For this review, take the finished solid that the model builds, in its own axes (mm). A direction names the side the tool comes from. Round coordinates to 2 decimals unless told otherwise and drop trailing zeros. Order: outer loops, then holes, each group sorted by start corner. A loop starts at its lowest first (then second) coordinate and runs counter-clockwise, first axis right, second up. Notation, with made-up numbers: M 39.5,-39.75 L 74.5,-39.75 A21 ccw 74.5,-30.75 Z; hole C 6.5,73 d8. An arc over 180 degrees is marked long. Write item = value, one per line. Start each with the question number.
from build123d import *

# Parameters (mm, degrees)
BOX_W           = 100
BOX_H           = 63
BOX_DEPTH       = 57
PAD_DEPTH       = 60
POCKET_DEPTH    = 60
SKETCH002_R     = 8.5
POCKET001_DEPTH = 5
SKETCH003_R     = 8.5
POCKET002_DEPTH = 5
SKETCH004_R     = 8.5
POCKET003_DEPTH = 5
SKETCH005_R     = 8.5
POCKET004_DEPTH = 5
SKETCH006_R     = 8.5
POCKET005_DEPTH = 5
SKETCH007_R     = 8.5
POCKET006_DEPTH = 5
SKETCH008_W     = 12
SKETCH008_H     = 3
PAD001_DEPTH    = 12
SKETCH009_W     = 12
SKETCH009_H     = 3
PAD002_DEPTH    = 12
SKETCH010_R     = 1.6
POCKET007_DEPTH = 5


with BuildPart() as cubo:
    # Box → Box (new body)
    with BuildSketch(Plane(origin=(-50, -62, -35), x_dir=(1, 0, 0), z_dir=(0, 0, 1))):
        with Locations((50, 31.5)):
            Rectangle(BOX_W, BOX_H)
    extrude(amount=BOX_DEPTH)


with BuildPart() as cut:
    # Sketch → Pad (new body)
    with BuildSketch(Plane.XZ):
        Polygon((0, 13.1372921726), (-24.1481456572, 6.666816045), (-41.8258151869, -11.0108534847), (-48.2962913145, -35.1589991419), (-41.8258151869, -59.3071447991), (-24.1481456572, -76.9848143288), (0, -83.4552904564), (24.1481456572, -76.9848143288), (41.8258151869, -59.3071447991), (48.2962913145, -35.1589991419), (41.8258151869, -11.0108534847), (24.1481456572, 6.666816045), align=None)
    extrude(amount=PAD_DEPTH)

    # Sketch001 (on Face13 of Pad) → Pocket (cut)
    with BuildSketch(Plane(origin=(0, 0, 0), x_dir=(1, 0, 0), z_dir=(0, 1, 0))):
        Polygon((0.2789274024, 81.4748360882), (23.1696976244, 75.2404980022), (40.0320556094, 58.422596), (46.1550508689, 34.895187618), (40.0872400093, 11.9994668326), (23.2933636529, -4.8586822764), (-0.3577352301, -11.1695458715), (-23.1458968596, -4.9360655293), (-40.0016837516, 11.8309415939), (-46.2963180976, 35.1693495985), (-39.9901052234, 58.5133129971), (-22.9100181577, 75.4141328541), align=None)
    extrude(amount=-POCKET_DEPTH, mode=Mode.SUBTRACT)

    # Sketch002 (on Face11 of Pocket) → Pocket001 (cut)
    with BuildSketch(Plane(origin=(-50.566479993, 0, -50.566479993), x_dir=(0.7071067812, 0, -0.7071067812), z_dir=(-0.7071067812, 0, -0.7071067812))):
        with Locations((24.861166713, 47)):
            Circle(SKETCH002_R)
        with Locations((24.861166713, 21)):
            Circle(SKETCH002_R)
    extrude(amount=-POCKET001_DEPTH, mode=Mode.SUBTRACT)

    # Sketch003 (on Face13 of Pocket001) → Pocket002 (cut)
    with BuildSketch(Plane(origin=(-20.8638226141, 0, -77.8648460359), x_dir=(0.9659258263, 0, -0.2588190451), z_dir=(-0.2588190451, 0, -0.9659258263))):
        with Locations((9.0998185847, 47)):
            Circle(SKETCH003_R)
        with Locations((9.0998185847, 21)):
            Circle(SKETCH003_R)
    extrude(amount=-POCKET002_DEPTH, mode=Mode.SUBTRACT)

    # Sketch004 (on Face14 of Pocket002) → Pocket003 (cut)
    with BuildSketch(Plane(origin=(20.8638226141, 0, -77.8648460359), x_dir=(0.9659258263, 0, 0.2588190451), z_dir=(0.2588190451, 0, -0.9659258263))):
        with Locations((-9.0998185847, 47)):
            Circle(SKETCH004_R)
        with Locations((-9.0998185847, 21)):
            Circle(SKETCH004_R)
    extrude(amount=-POCKET003_DEPTH, mode=Mode.SUBTRACT)

    # Sketch005 (on Face12 of Pocket003) → Pocket004 (cut)
    with BuildSketch(Plane(origin=(50.566479993, 0, -50.566479993), x_dir=(0.7071067812, 0, 0.7071067812), z_dir=(0.7071067812, 0, -0.7071067812))):
        with Locations((-24.861166713, 47)):
            Circle(SKETCH005_R)
        with Locations((-24.861166713, 21)):
            Circle(SKETCH005_R)
    extrude(amount=-POCKET004_DEPTH, mode=Mode.SUBTRACT)

    # Sketch006 (on Face10 of Pocket004) → Pocket005 (cut)
    with BuildSketch(Plane(origin=(53.8508030361, 0, -14.4292791853), x_dir=(0.2588190451, 0, 0.9659258263), z_dir=(0.9659258263, 0, -0.2588190451))):
        with Locations((-33.9609852976, 47)):
            Circle(SKETCH006_R)
        with Locations((-33.9609852976, 21)):
            Circle(SKETCH006_R)
    extrude(amount=-POCKET005_DEPTH, mode=Mode.SUBTRACT)

    # Sketch007 (on Face9 of Pocket005) → Pocket006 (cut)
    with BuildSketch(Plane(origin=(-53.8508030361, 0, -14.4292791853), x_dir=(0.2588190451, 0, -0.9659258263), z_dir=(-0.9659258263, 0, -0.2588190451))):
        with Locations((33.9609852976, 47)):
            Circle(SKETCH007_R)
        with Locations((33.9609852976, 21)):
            Circle(SKETCH007_R)
    extrude(amount=-POCKET006_DEPTH, mode=Mode.SUBTRACT)

    # Sketch008 (on Face14 of Pocket006) → Pad001 (join)
    with BuildSketch(Plane(origin=(20.8638226141, 0, -77.8648460359), x_dir=(0.9659258263, 0, 0.2588190451), z_dir=(0.2588190451, 0, -0.9659258263))):
        with Locations((-15.4992547125, 1.5258008155)):
            Rectangle(SKETCH008_W, SKETCH008_H)
    extrude(amount=PAD001_DEPTH)

    # Sketch009 (on Face13 of Pad001) → Pad002 (join)
    with BuildSketch(Plane(origin=(-20.8638226141, 0, -77.8648460359), x_dir=(0.9659258263, 0, -0.2588190451), z_dir=(-0.2588190451, 0, -0.9659258263))):
        with Locations((15.5166798155, 1.4931005082)):
            Rectangle(SKETCH009_W, SKETCH009_H)
    extrude(amount=PAD002_DEPTH)

    # Sketch010 (on Face42 of Pad002) → Pocket007 (cut)
    with BuildSketch(Plane.XZ.offset(3.0258008155)):
        with Locations((7.5046039895, -87.5720469825)):
            Circle(SKETCH010_R)
        with Locations((-7.1870487225, -87.7029523498)):
            Circle(SKETCH010_R)
    extrude(amount=-POCKET007_DEPTH, mode=Mode.SUBTRACT)

    # Cut: cut Cubo
    add(cubo.part, mode=Mode.SUBTRACT)


solid = cut.part
(1) For line 1 along X through (y, z) = (-3, -63.5); line 2 along X through (y, z) = (-38, -69); line 3 along Z through (x, y) = (29, -56), list the stretches that pass through material, from the lowest coordinate up.
(2) Draft analysis for pull direction X (two halves, no side actions). For faces 1 (the cylindrical face through (-44.599, -12.702, -45.202)), 2 (the flat face through (47, -30, -35)), 3 (the flat face through (13.22, -1.5, -86.04)), state which applies: released by +X, released by -X, zero draft, split by the parting line, or undercut.
(3) For faces 4 (the flat face through (-4, -60, -81)), 5 (the flat face through (-9, -2.993, -87)), 6 (the flat face through (29.609, -29.58, -68.818)), 7 (the flat face through (8.3, -3.026, -86)), list the 3-axis set-ups (+Z, -Z, +X, -X, +Y, -Y) from which the entire face can be reached by the end or side of a thin tool; tool diameter is ignored.
(4) We need section A-A, the plane y = -9.5. Write out the cut boundary in (x, z), then the cut area to 3 significant figures.
(5) Insertion check: pin 1 (1 mm diameter, centred on y = -31.5, z = -42.5, fed in from +X); pin 2 (2 mm diameter, centred on x = 3.5, y = -20.5, fed in from -Z); pin 3 (24 mm diameter, centred on x = -2.5, z = -69.5, fed in from +Y); pin 4 (10 mm diameter, centred on x = -22, z = -67, fed in from -Y). Each pin has a flat end and moves straight along its axis. Give the tip position at first contact, or say it passes through.
(6) We need section B-B, the plane z = -53.5. State how many separate pieces and enclosed holes the cut face has, then the cut area to 3 significant figures.
Values:
q1.line_1 = -37.63 to -34.95, 34.94 to 37.63
q1.line_2 = -32.13 to -29.39, 29.43 to 32.13
q1.line_3 = -72.13 to -69.43
q2.face_1 = undercut
q2.face_2 = zero draft
q2.face_3 = released by +X
q3.face_4 = +Z, -Z, +X, -X, -Y
q3.face_5 = -Z, -X, -Y
q3.face_6 = +Z, +Y, -Y
q3.face_7 = -Z, +X, -Y
q4.outline = M -48.3,-35.16 L -41.83,-59.31 L -24.15,-76.98 L 0,-83.46 L 24.15,-76.98 L 41.83,-59.31 L 48.3,-35.16 L 48.25,-35 L 46.13,-35 L 40.03,-58.42 L 23.17,-75.24 L 0.28,-81.47 L -22.91,-75.41 L -39.99,-58.51 L -46.3,-35.17 L -46.25,-35 L -48.25,-35 Z
q4.area = 285 mm²
q5.pin_1 = 46.46
q5.pin_2 = -82.79
q5.pin_3 = 0
q5.pin_4 = through
q6.separate_pieces = 6
q6.enclosed_holes = 0
q6.area = 162 mm²
